```python
from build123d import *

# Parameters (mm, degrees)
SKETCH1_R           = 255
BOSS_EXTRUDE1_DEPTH = 125
SHELL1_T            = -10
SKETCH3_W           = 120
SKETCH3_H           = 170
BOSS_EXTRUDE3_DEPTH = 20
SKETCH2_R           = 255
SKETCH2_R_2         = 250
BOSS_EXTRUDE2_DEPTH = 5
SKETCH5_W           = 110
SKETCH5_H           = 160
CUT_EXTRUDE1_DEPTH  = 15


with BuildPart() as part:
    # Sketch1 → Boss-Extrude1 (new body)
    with BuildSketch(Plane(origin=(0, 0, 0), x_dir=(1, 0, 0), z_dir=(0, 1, 0))):
        with Locations(Location((0, 0, 0), (0, 0, 270))):
            Circle(SKETCH1_R)
    extrude(amount=BOSS_EXTRUDE1_DEPTH)

    # Shell1
    shell1_openings = [part.faces().sort_by_distance(p)[0] for p in [
        (0, 125, 0),
    ]]
    offset(amount=SHELL1_T, openings=shell1_openings, kind=Kind.INTERSECTION)

    # Sketch3 → Boss-Extrude3 (add)
    with BuildSketch(Plane(origin=(0, 10, 0), x_dir=(1, 0, 0), z_dir=(0, 1, 0))):
        with Locations((0, 135)):
            Rectangle(SKETCH3_W, SKETCH3_H)
        Polygon((73.301270189, 26.961524227), (220.525588833, -58.038475773), (160.525588833, -161.961524227), (13.301270189, -76.961524227), align=None)
        Polygon((-13.301270189, -76.961524227), (-160.525588833, -161.961524227), (-220.525588833, -58.038475773), (-73.301270189, 26.961524227), align=None)
    extrude(amount=BOSS_EXTRUDE3_DEPTH)

    # Sketch2 → Boss-Extrude2 (add)
    with BuildSketch(Plane(origin=(0, 125, 0), x_dir=(1, 0, 0), z_dir=(0, 1, 0))):
        with Locations(Location((0, 0, 0), (0, 0, 270))):
            Circle(SKETCH2_R)
        with Locations(Location((0, 0, 0), (0, 0, 270))):
            Circle(SKETCH2_R_2, mode=Mode.SUBTRACT)
    extrude(amount=BOSS_EXTRUDE2_DEPTH)

    # Sketch5 → Cut-Extrude1 (cut)
    with BuildSketch(Plane(origin=(0, 30, 0), x_dir=(1, 0, 0), z_dir=(0, 1, 0))):
        Polygon((20.131397208, -75.131397208), (158.695461814, -155.131397208), (213.695461814, -59.868602792), (75.131397208, 20.131397208), align=None)
        with Locations((0, 135)):
            Rectangle(SKETCH5_W, SKETCH5_H)
        Polygon((-75.131397208, 20.131397208), (-213.695461814, -59.868602792), (-158.695461814, -155.131397208), (-20.131397208, -75.131397208), align=None)
    extrude(amount=-CUT_EXTRUDE1_DEPTH, mode=Mode.SUBTRACT)


solid = part.part
```
Geometry: final body of the model. Coordinates: model frame, mm. A direction names the side the tool comes from. Coordinates: 2 decimals unless noted, no trailing zeros. Order: outer loops, then holes, each group sorted by start corner. A loop starts at its lowest first (then second) coordinate and runs counter-clockwise, first axis right, second up. Notation, with made-up numbers: (40.5, -17) - (90.5, -17) arc R28 cw to (90.5, 10) - close; hole circle Ø9 at (52, 46). An arc over 180 degrees is marked (long way). Write each question's results on one line, items separated by ' | '.
1) Pin query (flat end, axial travel): pin 1 (3 mm diameter, centred on y = 77.5, z = 195, fed in from -X); pin 2 (12 mm diameter, centred on x = 152, z = 34, fed in from +Y); pin 3 (10 mm diameter, centred on x = 22, y = 20, fed in from +Z). Return the tip coordinate at first contact, or that it passes through.
Results list:
pin 1: x = -166.08 | pin 2: y = 15 | pin 3: z = 254.43
2) Section A-A, the plane y = 95. Return loops of the section in (x, z).
Results list:
outline: circle Ø510 at (0, 0); hole circle Ø490 at (0, 0)
3) Set-up query: faces 3 (the flat face through (-55, 23, -134)), 4 (the flat face through (-169, 130, 188)). Return all of +Z, -Z, +X, -X, +Y, -Y with unobstructed straight access to the full face (end or side cutting, diameter ignored); none if empty.
Results list:
face 3: +Y | face 4: +Z, -Z, +X, -X, +Y
4) Section D-D, the plane z = -130. Return loops of the section in (x, y), plus the area to 3 significant figures.
Results list:
outline: (-219.37, 0) - (219.37, 0) - (219.37, 130) - (213.54, 130) - (213.54, 125) - (207.67, 125) - (207.67, 10) - (60, 10) - (60, 30) - (55, 30) - (55, 15) - (-55, 15) - (-55, 30) - (-60, 30) - (-60, 10) - (-207.67, 10) - (-207.67, 125) - (-213.54, 125) - (-213.54, 130) - (-219.37, 130) - close | area: 7,890 mm^2
5) Pull-direction query (X, two-part tool) for faces 1 (the flat face through (4, 0, -4)), 2 (the flat face through (-90.4, 22.6, 115.7)); classes: pulls with the +X half, pulls with the -X half, needs draft (parallel to the pull), parting line crosses it, or undercut.
Results list:
face 1: needs draft | face 2: undercut
6) Line query: line 1 (X direction, y = 82, z = 0); line 2 (X direction, y = 27, z = 107); line 3 (Z direction, x = -133.5, y = 13). Output: solid intervals per line, ascending. Write a range as from..to.
Results list:
line 1: -255..-245, 245..255 | line 2: -231.46..-220.4, -192.26..-186.48, -75.33..-65.33, 65.33..75.33, 186.48..192.26, 220.4..231.46 | line 3: -217.26..-205.43, 7.79..146.36, 205.43..217.26
7) Section C-C, the plane x = 0. Return loops of the section in (y, z).
Results list:
outline: (0, -255) - (130, -255) - (130, -250) - (125, -250) - (125, -245) - (10, -245) - (10, -220) - (30, -220) - (30, -215) - (15, -215) - (15, -55) - (30, -55) - (30, -50) - (10, -50) - (10, 245) - (125, 245) - (125, 250) - (130, 250) - (130, 255) - (0, 255) - close
8) Section B-B, the plane z = 0. Return loops of the section in (x, y), plus the area to 3 significant figures.
Results list:
outline: (-255, 0) - (255, 0) - (255, 130) - (250, 130) - (250, 125) - (245, 125) - (245, 10) - (120, 10) - (120, 30) - (110, 30) - (110, 15) - (63.51, 15) - (63.51, 30) - (57.74, 30) - (57.74, 10) - (-57.74, 10) - (-57.74, 30) - (-63.51, 30) - (-63.51, 15) - (-110, 15) - (-110, 30) - (-120, 30) - (-120, 10) - (-245, 10) - (-245, 125) - (-250, 125) - (-250, 130) - (-255, 130) - close | area: 8,550 mm^2
